from build123d import *

# Parameters (mm, degrees)
BOSS_EXTRUDE1_DEPTH = 0.15
FILLET1_R           = 0.3
FILLET2_R           = 0.5
FILLET3_R           = 2


with BuildPart() as part:
    # Sketch1 → Boss-Extrude1 (new, symmetric)
    with BuildSketch(Plane.XY):
        Polygon((0, 0), (0.4, 0), (0.4, -0.6), (0.7, -0.6), (0.7, 0), (4.34307957, 0), (13.55, -6.5), (13.55, -9.5), (12.55, -11), (11.55, -9.5), (11.55, -7.5362203), (3, -1.5), (0, -1.5), align=None)
    extrude(amount=BOSS_EXTRUDE1_DEPTH, both=True)

    # Fillet1
    fillet1_edges = [part.edges().sort_by_distance(p)[0] for p in [
        (12.55, -11, 0),
    ]]
    fillet(fillet1_edges, radius=FILLET1_R)

    # Fillet2
    fillet2_edges = [part.edges().sort_by_distance(p)[0] for p in [
        (13.55, -9.5, 0),
        (11.55, -9.5, 0),
        (0, -1.5, 0),
    ]]
    fillet(fillet2_edges, radius=FILLET2_R)

    # Fillet3
    fillet3_edges = [part.edges().sort_by_distance(p)[0] for p in [
        (4.34307957, 0, 0),
        (13.55, -6.5, 0),
        (11.55, -7.5362203, 0),
        (3, -1.5, 0),
    ]]
    fillet(fillet3_edges, radius=FILLET3_R)


solid = part.part
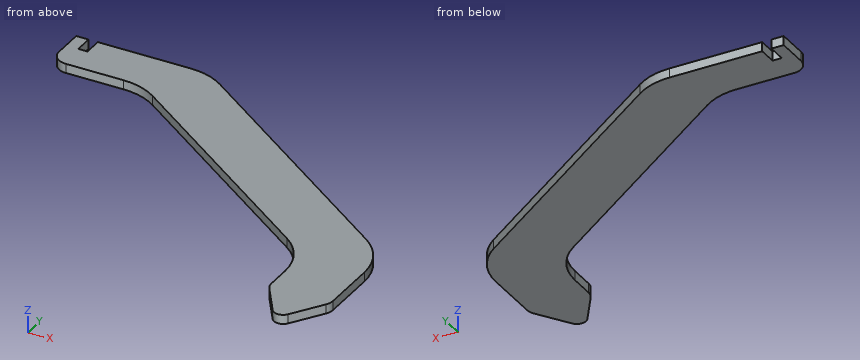
The model under review builds one solid part; all positions refer to its coordinate system, in mm. Coordinates: 2 decimals unless noted, no trailing zeros. Write each loop counter-clockwise with the first axis right and the second up, starting at its lowest first coordinate (ties: lowest second). Pieces come first, ordered by that corner, then holes. Notation, with made-up numbers: (8.5, -12.75) - (47.5, -12.75) arc R17 ccw to (47.5, 20.25) - close; hole circle Ø9 at (86, 65). An arc over 180 degrees is marked (long way). Answer as a JSON object with one key per item and string values. Group by question number.
1. Add section B-B (y = -8.75). Give the boundary of the cut face in (x, z).
2. Add section C-C (x = 5.5). Give the boundary of the cut face in (y, z), plus the area to 3 significant figures.
3. Add section A-A (z = -0.1). Give the boundary of the cut face in (x, y).
4. To check wall thickness, follow probe 1 along X at (y, z) = (-8.5, 0); probe 2 along Y at (x, z) = (2.25, 0.05). State the ranges of each line that lie inside material, in increasing order.
Findings:
{
 "1": {"outline": "(11.55, -0.15) - (13.55, -0.15) - (13.55, 0.15) - (11.55, 0.15) - close"},
 "2": {"outline": "(-3.26, -0.15) - (-0.82, -0.15) - (-0.82, 0.15) - (-3.26, 0.15) - close", "area": "0.734 mm²"},
 "3": {"outline": "(0, -1) arc R0.5 ccw to (0.5, -1.5) - (2.37, -1.5) arc R2 cw to (3.52, -1.87) - (10.7, -6.94) arc R2 cw to (11.55, -8.57) - (11.55, -9.35) arc R0.5 ccw to (11.63, -9.63) - (12.3, -10.63) arc R0.3 ccw to (12.8, -10.63) - (13.47, -9.63) arc R0.5 ccw to (13.55, -9.35) - (13.55, -7.54) arc R2 ccw to (12.7, -5.9) - (4.86, -0.37) arc R2 ccw to (3.71, 0) - (0.7, 0) - (0.7, -0.6) - (0.4, -0.6) - (0.4, 0) - (0, 0) - close"},
 "4": {"probe 1": "11.55 to 13.55", "probe 2": "-1.5 to 0"}
}
